Here's how the part is built. I have some questions about the finished solid (model axes, mm). A direction names the side the tool comes from. Round coordinates to 2 decimals unless told otherwise and drop trailing zeros. Write each loop counter-clockwise with the first axis right and the second up, starting at its lowest first coordinate (ties: lowest second). Pieces come first, ordered by that corner, then holes. Notation, with made-up numbers: (24, 3) -> (64, 3) arc R20 cw to (64, 20) -> close; hole circle Ø8 at (-7, 14). An arc over 180 degrees is marked (long way). Put each result on its own line as item: value. Start each with the question number.
1) We'd pull the mould along Z, two halves only. Please class faces 1 (the flat face through (15, -25, 22)), 2 (the flat face through (0, 25, 45)), 3 (the cylindrical face through (52.54, 4.21, 41.23)): released by +Z, released by -Z, zero draft, split by the parting line, or undercut.
2) I want a section at A-A, the plane y = 4.5. List the corners of the cut face in (x, z) for me.
3) Will these pins go through, and if not, where does the flat tip stop? P1, Ø11, axis at y = 24, z = 30, coming from the -X side; P2, Ø5.5, axis at y = 33.5, z = 2, coming from the -X side; P3, Ø5, axis at x = -20.5, y = -37.5, coming from the +Z side; P4, Ø5, axis at y = 25, z = 21.5, coming from the +X side.
4) Which directions (+Z, -Z, +X, -X, +Y, -Y) give clear straight access to the entire face, cutting with the end or side of a thin tool? Please do faces 4 (the flat face through (0, -20, 25)), 5 (the flat face through (51, 20, 16)), 6 (the flat face through (15, 25, 22)), 7 (the flat face through (0, -30, 25)).
5) If I drill on line 1 along Z through (x, y) = (-52.95, -5); line 2 along Y through (x, z) = (0, 33); line 3 along X through (y, z) = (24, 40.5), over which ranges is the centre line in solid material (lowest first)? Write a range as [from, to].
6) I want a section at C-C, the plane z = 33. List the corners of the cut face in (x, y) for me, then the cut area to 3 significant figures.
7) I want a section at D-D, the plane x = -39. List the corners of the cut face in (y, z) for me, then the cut area to 3 significant figures.
8) I want a section at B-B, the plane x = 0. List the corners of the cut face in (y, z) for me, then the cut area to 3 significant figures.
from build123d import *

# Parameters (mm, degrees)
F0_W      = 30
F0_H      = 100
F1_DEPTH  = 5
F2_W      = 30
F2_H      = 10
F3_DEPTH  = 40
F4_R      = 5
F5_R      = 2.5
F6_DEPTH  = 80.001
F7_W      = 40
F7_H      = 5
F8_DEPTH  = 25
F9_W      = 5
F9_H      = 40
F10_DEPTH = 40
F11_R     = 2.25
F12_DEPTH = 25


with BuildPart() as f1:
    # F0 (on Top) → F1 (new body)
    with BuildSketch(Plane.XY):
        with Locations((-15, 0)):
            Rectangle(F0_W, F0_H)
        with Locations((15, 0)):
            Rectangle(F0_W, F0_H)
    extrude(amount=F1_DEPTH)

    # F2 (on face) → F3 (join)
    with BuildSketch(Plane.XY.offset(5)):
        with Locations((0, 25)):
            Rectangle(F2_W, F2_H)
        with Locations((0, -25)):
            Rectangle(F2_W, F2_H)
    extrude(amount=F3_DEPTH)

    # F4
    f4_edges = [f1.edges().sort_by_distance(p)[0] for p in [
        (-15, -25, 45),
        (15, -25, 45),
        (-15, 25, 45),
        (15, 25, 45),
    ]]
    fillet(f4_edges, radius=F4_R)

    # F5 (on face) → F6 (cut, through all)
    with BuildSketch(Plane.XZ.offset(30)):
        with Locations((0, 40.5)):
            Circle(F5_R)
    extrude(amount=-F6_DEPTH, mode=Mode.SUBTRACT)

    # F7 (on face) → F8 (join)
    with BuildSketch(Plane.YZ.offset(30)):
        with Locations((0, 2.5)):
            Rectangle(F7_W, F7_H)
    extrude(amount=F8_DEPTH)

    # F9 (on face) → F10 (join)
    with BuildSketch(Plane.XY.offset(5)):
        with Locations((52.5, 0)):
            Rectangle(F9_W, F9_H)
    extrude(amount=F10_DEPTH)

    # F11 (on face) → F12 (cut)
    with BuildSketch(Plane.YZ.offset(55)):
        with Locations((-5, 39)):
            Circle(F11_R)
        with Locations((4.5, 39)):
            Circle(F11_R)
    extrude(amount=-F12_DEPTH, mode=Mode.SUBTRACT)

    # F15: F1 across plane


with BuildPart() as f1_1:
    add(f1.part)
    add(f1.part.mirror(Plane(origin=(0, 0, 5.5), x_dir=(0, -1, 0), z_dir=(-1, 0, 0))))


solid = f1_1.part
Findings:
1. face 1: zero draft
1. face 2: released by +Z
1. face 3: undercut
2. outline: (-55, 0) -> (55, 0) -> (55, 36.75) -> (50, 36.75) -> (50, 5) -> (-50, 5) -> (-50, 36.75) -> (-55, 36.75) -> close; (-55, 41.25) -> (-50, 41.25) -> (-50, 45) -> (-55, 45) -> close; (50, 41.25) -> (55, 41.25) -> (55, 45) -> (50, 45) -> close
3. P1: stops at x = -55
3. P2: stops at x = -30
3. P3: stops at z = 5
3. P4: stops at x = 15
4. face 4: +Z
4. face 5: +Z, -Z, +X, +Y
4. face 6: +Z, +X, +Y, -Y
4. face 7: +Z, +X, -X, -Y
5. line 1: z = [0, 36.75], [41.25, 45]
5. line 2: y = [-30, -20], [20, 30]
5. line 3: x = [-14.97, -2.5], [2.5, 14.97]
6. outline: (-55, -20) -> (-50, -20) -> (-50, 20) -> (-55, 20) -> close; (-15, -30) -> (15, -30) -> (15, -20) -> (-15, -20) -> close; (-15, 20) -> (15, 20) -> (15, 30) -> (-15, 30) -> close; (50, -20) -> (55, -20) -> (55, 20) -> (50, 20) -> close
6. area: 1,000 mm2
7. outline: (-20, 0) -> (20, 0) -> (20, 5) -> (-20, 5) -> close
7. area: 200 mm2
8. outline: (-50, 0) -> (50, 0) -> (50, 5) -> (30, 5) -> (30, 38) -> (20, 38) -> (20, 5) -> (-20, 5) -> (-20, 38) -> (-30, 38) -> (-30, 5) -> (-50, 5) -> close; (-30, 43) -> (-20, 43) -> (-20, 45) -> (-30, 45) -> close; (20, 43) -> (30, 43) -> (30, 45) -> (20, 45) -> close
8. area: 1,200 mm2
